Here's how the part is built. I have some questions about the finished solid (model axes, mm). A direction names the side the tool comes from. Coordinates: 2 decimals unless noted, no trailing zeros. Loops run counter-clockwise (first coordinate to the right, second up) from the corner with the lowest first, then second, coordinate; pieces in that order, holes last. Notation, with made-up numbers: (67.25, 28.25) -> (108.25, 28.25) arc R26 cw to (108.25, 61.25) -> close; hole circle Ø11 at (39.25, 2). An arc over 180 degrees is marked (long way). Answer as a JSON object with one key per item and string values. Group by question number.
Q1. I want a section at A-A on x = 50. Write out the boundary of the cut face in (y, z).
Q2. On a 3-axis mill with a long thin cutter (end or side, diameter ignored), from which of +Z, -Z, +X, -X, +Y, -Y can I reach the whole of each face in a straight line? I mean faces 1 (the flat face through (100, -1, 5)), 2 (the flat face through (-50, -10, 15)), 3 (the flat face through (-100, -1, 5)), 4 (the flat face through (-50, 10, 15)), 5 (the flat face through (-50, -8, 15)). Say none if no direction works.
Q3. I'm going to push flat-ended pins straight in: pin 1 (1.6 mm diameter, centred on y = -9.5, z = 15.5, fed in from -X); pin 2 (3 mm diameter, centred on x = -53, z = 14.5, fed in from -Y); pin 3 (1.6 mm diameter, centred on y = 8.5, z = 13.5, fed in from +X). Where does each tip first touch, or does it pass through?
Q4. I want a section at B-B on y = 0. Write out the boundary of the cut face in (x, z), then the cut area to 3 significant figures.
Q5. I need wall thicknesses on line 1 (Y direction, x = 50, z = 4.75); line 2 (Z direction, x = -42, y = 42); line 3 (Y direction, x = -38, z = 18.75). Which ranges of each line are inside material? Lowest first, please.
Q6. I want a section at C-C on x = -44. Write out the boundary of the cut face in (y, z), then the cut area to 3 significant figures.
Q7. Thinking about a two-plate mould opening in Y: for faces 6 (the cylindrical face through (51.847, -0.766, 4.93)), 7 (the flat face through (-50, 8, 15)), 8 (the flat face through (-1, 50, 5)), 9 (the flat face through (-1, -50, 5)), which applies, released by +Y, released by -Y, zero draft, split by the parting line, or undercut?
Q8. I want a section at D-D on y = -43. Write out the boundary of the cut face in (x, z).
```python
from build123d import *

# Parameters (mm, degrees)
SKETCH1_W           = 200
SKETCH1_H           = 100
SKETCH1_R           = 2
SKETCH1_W_2         = 40
SKETCH1_H_2         = 2
BOSS_EXTRUDE2_DEPTH = 10
SKETCH1_4_W         = 40
SKETCH1_4_H         = 2
BOSS_EXTRUDE3_DEPTH = 20


with BuildPart() as part:
    # Sketch1 → Boss-Extrude2 (new body)
    with BuildSketch(Plane.XY):
        Rectangle(SKETCH1_W, SKETCH1_H)
        with Locations((50, 0)):
            Circle(SKETCH1_R, mode=Mode.SUBTRACT)
        with Locations((-50, 9)):
            Rectangle(SKETCH1_W_2, SKETCH1_H_2, mode=Mode.SUBTRACT)
        with Locations((-50, -9)):
            Rectangle(SKETCH1_W_2, SKETCH1_H_2, mode=Mode.SUBTRACT)
    extrude(amount=BOSS_EXTRUDE2_DEPTH)

    # Sketch1_4 → Boss-Extrude3 (add)
    with BuildSketch(Plane.XY):
        with Locations((-50, 9)):
            Rectangle(SKETCH1_4_W, SKETCH1_4_H)
        with Locations((-50, -9)):
            Rectangle(SKETCH1_4_W, SKETCH1_4_H)
    extrude(amount=BOSS_EXTRUDE3_DEPTH)


solid = part.part
```
Result set:
{
 "1": {"outline": "(-50, 0) -> (-2, 0) -> (-2, 10) -> (-50, 10) -> close; (2, 0) -> (50, 0) -> (50, 10) -> (2, 10) -> close"},
 "2": {"face 1": "+Z, -Z, +X, +Y, -Y", "face 2": "+Z, +X, -X, -Y", "face 3": "+Z, -Z, -X, +Y, -Y", "face 4": "+Z, +X, -X, +Y", "face 5": "+Z, +X, -X"},
 "3": {"pin 1": "stops at x = -70", "pin 2": "stops at y = -10", "pin 3": "stops at x = -30"},
 "4": {"outline": "(-100, 0) -> (48, 0) -> (48, 10) -> (-100, 10) -> close; (52, 0) -> (100, 0) -> (100, 10) -> (52, 10) -> close", "area": "1,960 mm²"},
 "5": {"line 1": "y = -50 to -2, 2 to 50", "line 2": "z = 0 to 10", "line 3": "y = -10 to -8, 8 to 10"},
 "6": {"outline": "(-50, 0) -> (50, 0) -> (50, 10) -> (10, 10) -> (10, 20) -> (8, 20) -> (8, 10) -> (-8, 10) -> (-8, 20) -> (-10, 20) -> (-10, 10) -> (-50, 10) -> close", "area": "1,040 mm²"},
 "7": {"face 6": "undercut", "face 7": "undercut", "face 8": "released by +Y", "face 9": "released by -Y"},
 "8": {"outline": "(-100, 0) -> (100, 0) -> (100, 10) -> (-100, 10) -> close"}
}
